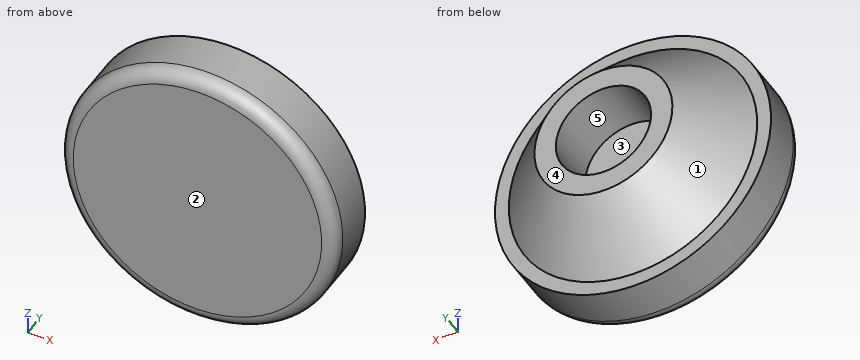
from build123d import *

# Parameters (mm, degrees)
ESBO_O1_R                = 5
RESSALTO_EXTRUS_O1_DEPTH = 2
ESBO_O2_R                = 2.5
RESSALTO_EXTRUS_O2_DEPTH = 2
ESBO_O3_R                = 1.725
CORTE_EXTRUS_O1_DEPTH    = 2
CHANFRO1_SIZE            = 2
FILETE1_R                = 0.5


with BuildPart() as part:
    # Esboço1 → Ressalto-extrusão1 (new body)
    with BuildSketch(Plane(origin=(0, 0, 0), x_dir=(1, 0, 0), z_dir=(0, 1, 0))):
        with Locations(Location((0, 0, 0), (0, 0, 270))):
            Circle(ESBO_O1_R)
    extrude(amount=RESSALTO_EXTRUS_O1_DEPTH)

    # Esboço2 → Ressalto-extrusão2 (add)
    with BuildSketch(Plane(origin=(0, 2, 0), x_dir=(1, 0, 0), z_dir=(0, 1, 0))):
        with Locations(Location((0, 0, 0), (0, 0, 270))):
            Circle(ESBO_O2_R)
    extrude(amount=RESSALTO_EXTRUS_O2_DEPTH)

    # Esboço3 → Corte-extrusão1 (cut)
    with BuildSketch(Plane(origin=(0, 4, 0), x_dir=(1, 0, 0), z_dir=(0, 1, 0))):
        with Locations(Location((0, 0, 0), (0, 0, 270))):
            Circle(ESBO_O3_R)
    extrude(amount=-CORTE_EXTRUS_O1_DEPTH, mode=Mode.SUBTRACT)

    # Chanfro1
    chanfro1_edges = [part.edges().sort_by_distance(p)[0] for p in [
        (0, 2, -2.5),
    ]]
    chamfer(chanfro1_edges, length=CHANFRO1_SIZE - 0.0001)  # a hair under: the kernel refuses the full size

    # Filete1
    filete1_edges = [part.edges().sort_by_distance(p)[0] for p in [
        (0, 0, -5),
    ]]
    fillet(filete1_edges, radius=FILETE1_R)


solid = part.part
Here's how the part is built. I have some questions about the finished solid (model axes, mm). Face numbers are marked on the shaded views. A direction names the side the tool comes from. Round coordinates to 2 decimals unless told otherwise and drop trailing zeros. Order: outer loops, then holes, each group sorted by start corner. A loop starts at its lowest first (then second) coordinate and runs counter-clockwise, first axis right, second up. Notation, with made-up numbers: (5.25, 78.25) -> (20.25, 78.25) arc R27 ccw to (20.25, 104.25) -> close; hole circle Ø3 at (56, 61). An arc over 180 degrees is marked (long way). Return JSON: item names as keys, results as strings.
Q1. I need wall thicknesses on line 1 along Y through (x, z) = (0.75, -1.5); line 2 along X through (y, z) = (2.9, 1.5); line 3 along X through (y, z) = (3.6, 0) (3 decimals). Which ranges of each line are inside material? Lowest first, please. Write a range as from..to.
Filled sheet:
{"line 1": "y = 0..2", "line 2": "x = -3.27..-0.85, 0.85..3.27", "line 3": "x = -2.9..-1.725, 1.725..2.9"}
Q2. If we section it at D-D on y = 2.6: List the corners of the cut face in (x, z) for me (3 decimals), plus the area to 3 significant figures.
Filled sheet:
{"outline": "circle Ø7.8 at (0, 0); hole circle Ø3.45 at (0, 0)", "area": "38.4 mm^2"}
Q3. If we mould it in two halves opening along X, with no side actions, what happens to the marked faces 1, 2 and 3? For each: released by +X, released by -X, zero draft, split by the parting line, or undercut.
Filled sheet:
{"face 1": "split by the parting line", "face 2": "zero draft", "face 3": "undercut"}
Q4. If we section it at C-C on y = 1.3: List the corners of the cut face in (x, z) for me, plus the area to 3 significant figures.
Filled sheet:
{"outline": "circle Ø10 at (0, 0)", "area": "78.5 mm^2"}
Q5. Which directions (+Z, -Z, +X, -X, +Y, -Y) give clear straight access to the entire face, cutting with the end or side of a thin tool? Please do the marked faces 4 and 5.
Filled sheet:
{"face 4": "+Z, -Z, +X, -X, +Y", "face 5": "+Y"}
Q6. For pin 1 Ø1 at (x, z) = (1, 0) entering from +Y; pin 2 Ø2 at (x, y) = (-1.5, 1.5) entering from -Z; pin 3 Ø1.5 at (x, z) = (3.5, 0) entering from +Y, each with a flat end and sliding along its axis, tell me the tip position at first contact or that it passes through.
Filled sheet:
{"pin 1": "stops at y = 2", "pin 2": "stops at z = -4.97", "pin 3": "stops at y = 3.75"}
